Autodesk Inventor part; units mm, degrees
ref_plane "YZ Plane" through (0, 0, 0) normal (1, 0, 0) x (0, 1, 0)
ref_plane "XZ Plane" through (0, 0, 0) normal (0, 1, 0) x (-1, 0, 0)
ref_plane "XY Plane" through (0, 0, 0) normal (0, 0, 1) x (1, 0, 0)
sketch "スケッチ1" plane through (0, 0, 0) normal (0, 1, 0) x (-1, 0, 0)
  line L0 (-5.6, 0) -> (5.6, 0)
  line L1 (5.6, 0) -> (5.6, -2.2)
  line L2 (5.6, -2.2) -> (8.4, -2.2)
  line L3 (8.4, -2.2) -> (8.4, -5.2)
  line L4 (8.4, -5.2) -> (4.6551, -5.2)
  line L5 (4.6551, -5.2) -> (3.4551, -3.1215)
  line L6 (3.4551, -3.1215) -> (-3.4551, -3.1215)
  line L7 (-3.4551, -3.1215) -> (-4.6551, -5.2)
  line L8 (-4.6551, -5.2) -> (-8.4, -5.2)
  line L9 (-8.4, -5.2) -> (-8.4, -2.2)
  line L10 (-8.4, -2.2) -> (-5.6, -2.2)
  line L11 (-5.6, -2.2) -> (-5.6, 0)
  point P0 (0, 0)
  point P1 (0, 0)
  point P2 (0, -3.1215)
  dimension "d0" = 11.2
  dimension "d1" = 5.2
  dimension "d2" = 16.8
  dimension "d3" = 120
  dimension "d4" = 120
  dimension "d5" = 3
extrude "押し出し1" add sketch "スケッチ1" along normal blind 50
chamfer "面取り1" [suppressed]
chamfer "面取り2" distance 1 angle 45 4 edges at (8.4, 0, -3.7) (-8.4, 0, -3.7) (8.4, 50, -3.7) (-8.4, 50, -3.7)
chamfer "面取り3" distance 0.3 angle 45 4 edges at (-8.4, 25, -2.2) (-8.4, 25, -5.2) (8.4, 25, -5.2) (8.4, 25, -2.2)
sketch "スケッチ2" plane through (-5.6, 0, 0) normal (0, 0, 1) x (1, 0, 0)
  line L0 (5.6, 10) -> (5.6, 40) construction
  line L1 (13.7, 49.3) -> (13.7, 0.7) construction
  line L2 (0, 0) -> (11.2, 0) construction
  point P0 (5.6, 0)
  point P1 (5.6, 25)
  point P2 (13.7, 25)
  point P3 (5.6, 0)
  dimension "d17" = 30
hole "穴1" at (0, 10, 0) at (0, 40, 0) direction (0, 0, -1) diameter 3.242 end through all
properties part number "MR-20CS" material "ポリエチレン、高密度"
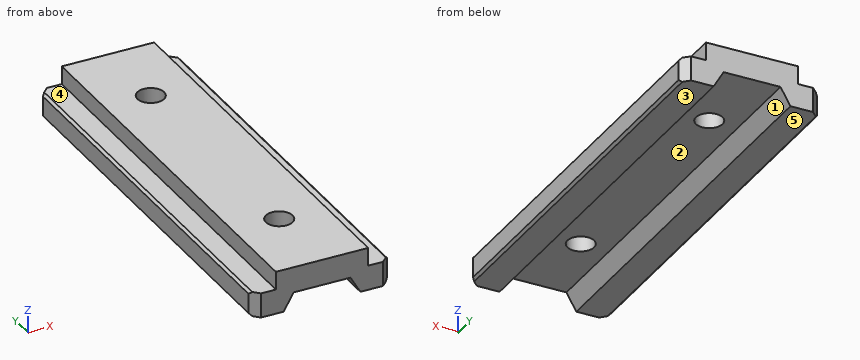
The listing builds one solid part. Answer for the finished solid, in the listing's coordinates (mm). Face numbers are marked on the shaded views. A direction names the side the tool comes from. Give positions to 0.01 mm unless a question says otherwise; leave off trailing zeros. Order: outer loops, then holes, each group sorted by start corner. A loop starts at its lowest first (then second) coordinate and runs counter-clockwise, first axis right, second up. Notation, with made-up numbers: (53.5, 88) -> (94.5, 88) arc R5 ccw to (94.5, 93) -> close; hole circle Ø11 at (-18.5, -3.75). An arc over 180 degrees is marked (long way). Answer as CSV lines item,"result". Start each with the question number.
Q1. Given pin 1 (3.5 mm diameter, centred on x = 0, y = 10, fed in from -Z); pin 2 (1.9 mm diameter, centred on x = 0, y = 40, fed in from -Z); pin 3 (3 mm diameter, centred on x = -7.5, y = 20.5, fed in from +Z); pin 4 (1.8 mm diameter, centred on y = 20.5, z = -1.5, fed in from -X), each flat-ended and moving along its own axis, determine where each tip first touches the part or whether it passes through.
Q2. Find the intervals of material crossed by L1, parallel to Y at x = 0, z = -2.05; L2, parallel to X at y = 10, z = -1.1; L3, parallel to Z at x = 1.5, y = 38.5, in increasing order.
Q3. A cutting plane is placed at B-B (y = 40). Determine the outline of the cut face in (x, z).
Q4. A cutting plane is placed at A-A (x = 0). Determine the outline of the cut face in (y, z), then the cut area to 3 significant figures.
Q5. Which of the six approach directions +Z, -Z, +X, -X, +Y, -Y give full straight-line access (tool end or side, diameter ignored) to the marked faces 4 and 5?
Q6. A cutting plane is placed at C-C (y = 25). Determine the outline of the cut face in (x, z).
Q7. Determine the mould class of the marked faces 1, 2 and 3 for opening direction X: pulls with the +X half, pulls with the -X half, needs draft (parallel to the pull), parting line crosses it, or undercut.
Results found:
1,pin 1,"z = -3.12"
1,pin 2,"through"
1,pin 3,"z = -2.2"
1,pin 4,"x = -8.3"
2,L1,"0 to 8.38, 11.62 to 38.38, 41.62 to 50"
2,L2,"-5.6 to -1.62, 1.62 to 5.6"
2,L3,"-3.12 to 0"
3,outline,"(-8.4, -4.9) -> (-8.1, -5.2) -> (-4.66, -5.2) -> (-3.46, -3.12) -> (-1.62, -3.12) -> (-1.62, 0) -> (-5.6, 0) -> (-5.6, -2.2) -> (-8.1, -2.2) -> (-8.4, -2.5) -> close; (1.62, -3.12) -> (3.46, -3.12) -> (4.66, -5.2) -> (8.1, -5.2) -> (8.4, -4.9) -> (8.4, -2.5) -> (8.1, -2.2) -> (5.6, -2.2) -> (5.6, 0) -> (1.62, 0) -> close"
4,outline,"(0, -3.12) -> (8.38, -3.12) -> (8.38, 0) -> (0, 0) -> close; (11.62, -3.12) -> (38.38, -3.12) -> (38.38, 0) -> (11.62, 0) -> close; (41.62, -3.12) -> (50, -3.12) -> (50, 0) -> (41.62, 0) -> close"
4,area,"136 mm2"
5,face 4,"+Z, -X, +Y, -Y"
5,face 5,"-Z, +X, -X, +Y, -Y"
6,outline,"(-8.4, -4.9) -> (-8.1, -5.2) -> (-4.66, -5.2) -> (-3.46, -3.12) -> (3.46, -3.12) -> (4.66, -5.2) -> (8.1, -5.2) -> (8.4, -4.9) -> (8.4, -2.5) -> (8.1, -2.2) -> (5.6, -2.2) -> (5.6, 0) -> (-5.6, 0) -> (-5.6, -2.2) -> (-8.1, -2.2) -> (-8.4, -2.5) -> close"
7,face 1,"undercut"
7,face 2,"undercut"
7,face 3,"needs draft"
